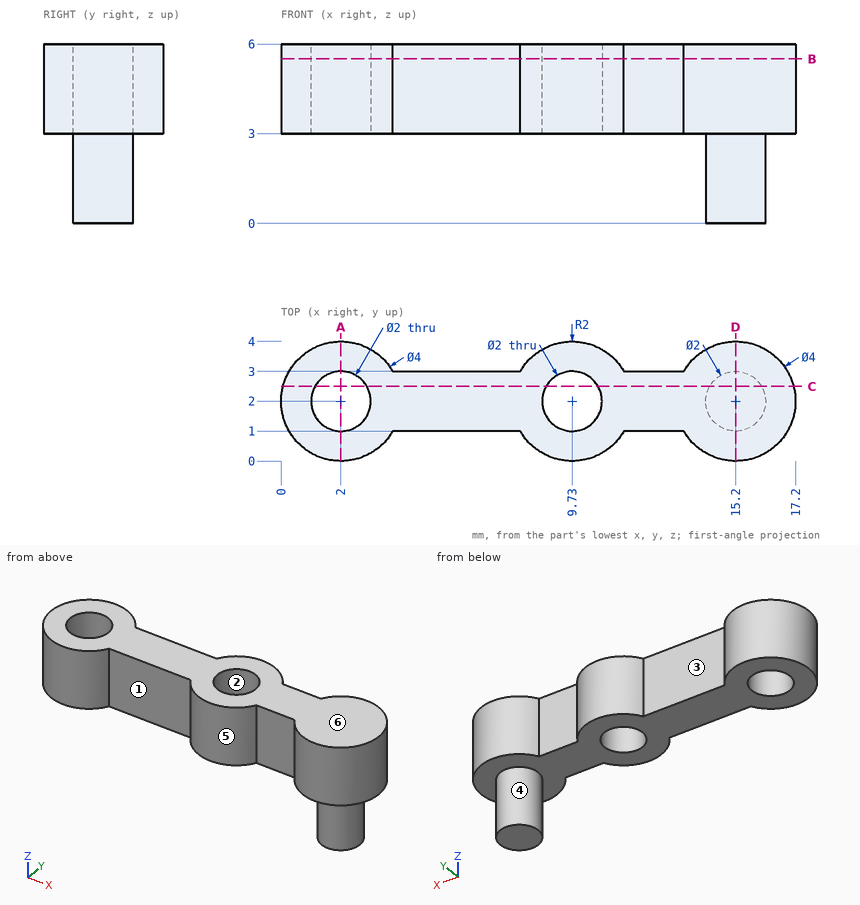
Job drawing, mm, ordinate dimensions from the low corner. One solid piece. A direction names the side the tool comes from. Coordinates: 2 decimals unless noted, no trailing zeros. Order: outer loops, then holes, each group sorted by start corner. A loop starts at its lowest first (then second) coordinate and runs counter-clockwise, first axis right, second up. Notation, with made-up numbers: (59.25, -28.75) - (91.25, -28.75) arc R21 ccw to (91.25, 0.25) - close; hole circle Ø10 at (15, 8). An arc over 180 degrees is marked (long way). Return JSON: item names as keys, results as strings. Group by question number.
1) Mould opens along X. For the marked faces 4, 5 and 6 say: released by +X, released by -X, zero draft, split by the parting line, or undercut.
2) Saw through at C-C, the plane y = 2.5. Write the cut outline in (x, z).
3) Flat gauge pins, fed straight in: P1, Ø1.6, axis at x = 12, z = 5, coming from the +Y side; P2, Ø1.6, axis at x = 12.5, z = 4, coming from the -Y side; P3, Ø0.9, axis at x = 6.5, z = 4.5, coming from the +Y side. Where does each tip first touch, or does it go through?
4) Saw through at D-D, the plane x = 15.2. Write the cut outline in (y, z), plus the area to 3 significant figures.
5) Saw through at A-A, the plane x = 2. Write the cut outline in (y, z).
6) Saw through at B-B, the plane z = 5.5. Write the cut outline in (x, y).
7) Tool access for the marked faces 1, 2 and 3: list every direction of +Z, -Z, +X, -X, +Y, -Y with a clear straight run to the whole face (end or side of a thin tool).
8) Probe line 1 (Y direction, x = 9.73, z = 4.2); line 2 (X direction, y = 0.7, z = 5.55); line 3 (X direction, y = 2.5, z = 4.65). List the from-to ranges inside material, lowest first. Write a range as from..to.
Values found:
{
 "1": {"face 4": "split by the parting line", "face 5": "undercut", "face 6": "zero draft"},
 "2": {"outline": "(0.06, 3) - (1.13, 3) - (1.13, 6) - (0.06, 6) - close; (2.87, 3) - (8.86, 3) - (8.86, 6) - (2.87, 6) - close; (10.6, 3) - (14.33, 3) - (14.33, 0) - (16.07, 0) - (16.07, 3) - (17.14, 3) - (17.14, 6) - (10.6, 6) - close"},
 "3": {"P1": "stops at y = 3.36", "P2": "stops at y = 1", "P3": "stops at y = 3"},
 "4": {"outline": "(0, 3) - (1, 3) - (1, 0) - (3, 0) - (3, 3) - (4, 3) - (4, 6) - (0, 6) - close", "area": "18.0 mm²"},
 "5": {"outline": "(0, 3) - (1, 3) - (1, 6) - (0, 6) - close; (3, 3) - (4, 3) - (4, 6) - (3, 6) - close"},
 "6": {"outline": "(3.73, 1) - (8, 1) arc R2 ccw to (11.46, 1) - (13.47, 1) arc R2 ccw (long way) to (13.47, 3) - (11.46, 3) arc R2 ccw to (8, 3) - (3.73, 3) arc R2 ccw (long way) to start; hole circle Ø2 at (2, 2); hole circle Ø2 at (9.73, 2)"},
 "7": {"face 1": "+Z, -Z, -Y", "face 2": "+Z, -Z", "face 3": "+Z, -Z, +Y"},
 "8": {"line 1": "y = 0..1, 3..4", "line 2": "x = 0.48..3.52, 8.21..11.25, 13.68..16.72", "line 3": "x = 0.06..1.13, 2.87..8.86, 10.6..17.14"}
}
